```python
from build123d import *

# Parameters (mm, degrees)
BASE_DEPTH                = 5
ESQUISSE3_R               = 2
ESQUISSE3_W               = 65
ESQUISSE3_H               = 30
ENL_V_MAT_EXTRU_1_DEPTH   = 6
CONG_1_R                  = 3
PER_AGE_POUR_BILLES_REACH = 7
ESQUISSE6_R               = 2
ESQUISSE6_R_2             = 10.5
PER_AGE_POUR_PROFIL_REACH = 7
ESQUISSE8_R               = 3
ESQUISSE10_R              = 2
ENL_V_MAT_EXTRU_3_DEPTH   = 6


with BuildPart() as part:
    # Esquisse1 → Base (new body)
    with BuildSketch(Plane.XY):
        Polygon((0, 0), (-130, 0), (-154.748737342, 24.748737342), (-154.748737342, 244.748737342), (-130, 269.497474683), (0, 269.497474683), (24.748737342, 244.748737342), (24.748737342, 24.748737342), align=None)
    extrude(amount=BASE_DEPTH)

    # Esquisse3 → Enlèv. mat.-Extru.1 (cut, through all)
    with BuildSketch(Plane(origin=(0, 0, 0), x_dir=(-1, 0, 0), z_dir=(0, 0, -1))):
        with Locations((30, 45)):
            Circle(ESQUISSE3_R)
        with Locations((100, 45)):
            Circle(ESQUISSE3_R)
        with Locations((100, 224.497474683)):
            Circle(ESQUISSE3_R)
        with Locations((30, 224.497474683)):
            Circle(ESQUISSE3_R)
        Polygon((107, 0), (107, 20), (83, 20), (83, 45.5), (47, 45.5), (47, 20), (23, 20), (23, 0), align=None)
        Polygon((23, 269.497474683), (107, 269.497474683), (107, 249.497474683), (83, 249.497474683), (83, 223.997474683), (47, 223.997474683), (47, 249.497474683), (23, 249.497474683), align=None)
        with Locations((65, 199.497474683)):
            Rectangle(ESQUISSE3_W, ESQUISSE3_H)
        with Locations((65, 70)):
            Rectangle(ESQUISSE3_W, ESQUISSE3_H)
    extrude(amount=-ENL_V_MAT_EXTRU_1_DEPTH, mode=Mode.SUBTRACT)

    # Congé1
    cong_1_edges = [part.edges().sort_by_distance(p)[0] for p in [
        (0, 0, 2.5),
        (-130, 0, 2.5),
        (-154.748737342, 24.748737342, 2.5),
        (-154.748737342, 244.748737342, 2.5),
        (-130, 269.497474683, 2.5),
        (0, 269.497474683, 2.5),
        (24.748737342, 244.748737342, 2.5),
        (24.748737342, 24.748737342, 2.5),
        (-23, 249.497474683, 2.5),
        (-23, 269.497474683, 2.5),
        (-107, 269.497474683, 2.5),
        (-107, 249.497474683, 2.5),
        (-83, 249.497474683, 2.5),
        (-83, 223.997474683, 2.5),
        (-47, 223.997474683, 2.5),
        (-47, 249.497474683, 2.5),
        (-107, 0, 2.5),
        (-23, 0, 2.5),
        (-23, 20, 2.5),
        (-47, 20, 2.5),
        (-47, 45.5, 2.5),
        (-83, 45.5, 2.5),
        (-83, 20, 2.5),
        (-107, 20, 2.5),
    ]]
    fillet(cong_1_edges, radius=CONG_1_R)

    # Esquisse6 → Perçage pour billes (cut, up to next)
    with BuildSketch(Plane.XY.offset(5), mode=Mode.PRIVATE) as per_age_pour_billes_sk1:
        with Locations((-142, 55)):
            Circle(ESQUISSE6_R)
    per_age_pour_billes_tool1 = extrude(per_age_pour_billes_sk1.sketch, amount=-PER_AGE_POUR_BILLES_REACH, mode=Mode.PRIVATE) & part.part
    add(per_age_pour_billes_tool1.solids().sort_by_distance((-142, 55, 5))[0], mode=Mode.SUBTRACT)
    # Esquisse6 → Perçage pour billes (cut, up to next)
    with BuildSketch(Plane.XY.offset(5), mode=Mode.PRIVATE) as per_age_pour_billes_sk2:
        with Locations((-142, 85)):
            Circle(ESQUISSE6_R)
    per_age_pour_billes_tool2 = extrude(per_age_pour_billes_sk2.sketch, amount=-PER_AGE_POUR_BILLES_REACH, mode=Mode.PRIVATE) & part.part
    add(per_age_pour_billes_tool2.solids().sort_by_distance((-142, 85, 5))[0], mode=Mode.SUBTRACT)
    # Esquisse6 → Perçage pour billes (cut, up to next)
    with BuildSketch(Plane.XY.offset(5), mode=Mode.PRIVATE) as per_age_pour_billes_sk3:
        with Locations((-142, 70)):
            Circle(ESQUISSE6_R_2)
    per_age_pour_billes_tool3 = extrude(per_age_pour_billes_sk3.sketch, amount=-PER_AGE_POUR_BILLES_REACH, mode=Mode.PRIVATE) & part.part
    add(per_age_pour_billes_tool3.solids().sort_by_distance((-142, 70, 5))[0], mode=Mode.SUBTRACT)
    # Esquisse6 → Perçage pour billes (cut, up to next)
    with BuildSketch(Plane.XY.offset(5), mode=Mode.PRIVATE) as per_age_pour_billes_sk4:
        with Locations((-142, 214.497474683)):
            Circle(ESQUISSE6_R)
    per_age_pour_billes_tool4 = extrude(per_age_pour_billes_sk4.sketch, amount=-PER_AGE_POUR_BILLES_REACH, mode=Mode.PRIVATE) & part.part
    add(per_age_pour_billes_tool4.solids().sort_by_distance((-142, 214.497475, 5))[0], mode=Mode.SUBTRACT)
    # Esquisse6 → Perçage pour billes (cut, up to next)
    with BuildSketch(Plane.XY.offset(5), mode=Mode.PRIVATE) as per_age_pour_billes_sk5:
        with Locations((-142, 184.497474683)):
            Circle(ESQUISSE6_R)
    per_age_pour_billes_tool5 = extrude(per_age_pour_billes_sk5.sketch, amount=-PER_AGE_POUR_BILLES_REACH, mode=Mode.PRIVATE) & part.part
    add(per_age_pour_billes_tool5.solids().sort_by_distance((-142, 184.497475, 5))[0], mode=Mode.SUBTRACT)
    # Esquisse6 → Perçage pour billes (cut, up to next)
    with BuildSketch(Plane.XY.offset(5), mode=Mode.PRIVATE) as per_age_pour_billes_sk6:
        with Locations((-142, 199.497474683)):
            Circle(ESQUISSE6_R_2)
    per_age_pour_billes_tool6 = extrude(per_age_pour_billes_sk6.sketch, amount=-PER_AGE_POUR_BILLES_REACH, mode=Mode.PRIVATE) & part.part
    add(per_age_pour_billes_tool6.solids().sort_by_distance((-142, 199.497475, 5))[0], mode=Mode.SUBTRACT)
    # Esquisse6 → Perçage pour billes (cut, up to next)
    with BuildSketch(Plane.XY.offset(5), mode=Mode.PRIVATE) as per_age_pour_billes_sk7:
        with Locations((12, 55)):
            Circle(ESQUISSE6_R)
    per_age_pour_billes_tool7 = extrude(per_age_pour_billes_sk7.sketch, amount=-PER_AGE_POUR_BILLES_REACH, mode=Mode.PRIVATE) & part.part
    add(per_age_pour_billes_tool7.solids().sort_by_distance((12, 55, 5))[0], mode=Mode.SUBTRACT)
    # Esquisse6 → Perçage pour billes (cut, up to next)
    with BuildSketch(Plane.XY.offset(5), mode=Mode.PRIVATE) as per_age_pour_billes_sk8:
        with Locations((12, 184.497474683)):
            Circle(ESQUISSE6_R)
    per_age_pour_billes_tool8 = extrude(per_age_pour_billes_sk8.sketch, amount=-PER_AGE_POUR_BILLES_REACH, mode=Mode.PRIVATE) & part.part
    add(per_age_pour_billes_tool8.solids().sort_by_distance((12, 184.497475, 5))[0], mode=Mode.SUBTRACT)
    # Esquisse6 → Perçage pour billes (cut, up to next)
    with BuildSketch(Plane.XY.offset(5), mode=Mode.PRIVATE) as per_age_pour_billes_sk9:
        with Locations((12, 214.497474683)):
            Circle(ESQUISSE6_R)
    per_age_pour_billes_tool9 = extrude(per_age_pour_billes_sk9.sketch, amount=-PER_AGE_POUR_BILLES_REACH, mode=Mode.PRIVATE) & part.part
    add(per_age_pour_billes_tool9.solids().sort_by_distance((12, 214.497475, 5))[0], mode=Mode.SUBTRACT)
    # Esquisse6 → Perçage pour billes (cut, up to next)
    with BuildSketch(Plane.XY.offset(5), mode=Mode.PRIVATE) as per_age_pour_billes_sk10:
        with Locations((12, 85)):
            Circle(ESQUISSE6_R)
    per_age_pour_billes_tool10 = extrude(per_age_pour_billes_sk10.sketch, amount=-PER_AGE_POUR_BILLES_REACH, mode=Mode.PRIVATE) & part.part
    add(per_age_pour_billes_tool10.solids().sort_by_distance((12, 85, 5))[0], mode=Mode.SUBTRACT)
    # Esquisse6 → Perçage pour billes (cut, up to next)
    with BuildSketch(Plane.XY.offset(5), mode=Mode.PRIVATE) as per_age_pour_billes_sk11:
        with Locations((12, 70)):
            Circle(ESQUISSE6_R_2)
    per_age_pour_billes_tool11 = extrude(per_age_pour_billes_sk11.sketch, amount=-PER_AGE_POUR_BILLES_REACH, mode=Mode.PRIVATE) & part.part
    add(per_age_pour_billes_tool11.solids().sort_by_distance((12, 70, 5))[0], mode=Mode.SUBTRACT)
    # Esquisse6 → Perçage pour billes (cut, up to next)
    with BuildSketch(Plane.XY.offset(5), mode=Mode.PRIVATE) as per_age_pour_billes_sk12:
        with Locations((12, 199.497474683)):
            Circle(ESQUISSE6_R_2)
    per_age_pour_billes_tool12 = extrude(per_age_pour_billes_sk12.sketch, amount=-PER_AGE_POUR_BILLES_REACH, mode=Mode.PRIVATE) & part.part
    add(per_age_pour_billes_tool12.solids().sort_by_distance((12, 199.497475, 5))[0], mode=Mode.SUBTRACT)

    # Esquisse8 → Perçage pour profilé (cut, up to next)
    with BuildSketch(Plane.XY.offset(5), mode=Mode.PRIVATE) as per_age_pour_profil_sk1:
        with Locations((-118, 11)):
            Circle(ESQUISSE8_R)
    per_age_pour_profil_tool1 = extrude(per_age_pour_profil_sk1.sketch, amount=-PER_AGE_POUR_PROFIL_REACH, mode=Mode.PRIVATE) & part.part
    add(per_age_pour_profil_tool1.solids().sort_by_distance((-118, 11, 5))[0], mode=Mode.SUBTRACT)
    # Esquisse8 → Perçage pour profilé (cut, up to next)
    with BuildSketch(Plane.XY.offset(5), mode=Mode.PRIVATE) as per_age_pour_profil_sk2:
        with Locations((-118, 258.497474683)):
            Circle(ESQUISSE8_R)
    per_age_pour_profil_tool2 = extrude(per_age_pour_profil_sk2.sketch, amount=-PER_AGE_POUR_PROFIL_REACH, mode=Mode.PRIVATE) & part.part
    add(per_age_pour_profil_tool2.solids().sort_by_distance((-118, 258.497475, 5))[0], mode=Mode.SUBTRACT)
    # Esquisse8 → Perçage pour profilé (cut, up to next)
    with BuildSketch(Plane.XY.offset(5), mode=Mode.PRIVATE) as per_age_pour_profil_sk3:
        with Locations((-12, 258.497474683)):
            Circle(ESQUISSE8_R)
    per_age_pour_profil_tool3 = extrude(per_age_pour_profil_sk3.sketch, amount=-PER_AGE_POUR_PROFIL_REACH, mode=Mode.PRIVATE) & part.part
    add(per_age_pour_profil_tool3.solids().sort_by_distance((-12, 258.497475, 5))[0], mode=Mode.SUBTRACT)
    # Esquisse8 → Perçage pour profilé (cut, up to next)
    with BuildSketch(Plane.XY.offset(5), mode=Mode.PRIVATE) as per_age_pour_profil_sk4:
        with Locations((-12, 11)):
            Circle(ESQUISSE8_R)
    per_age_pour_profil_tool4 = extrude(per_age_pour_profil_sk4.sketch, amount=-PER_AGE_POUR_PROFIL_REACH, mode=Mode.PRIVATE) & part.part
    add(per_age_pour_profil_tool4.solids().sort_by_distance((-12, 11, 5))[0], mode=Mode.SUBTRACT)

    # Esquisse10 → Enlèv. mat.-Extru.3 (cut, through all)
    with BuildSketch(Plane.XY.offset(5)):
        with Locations((-97, 174.497474683)):
            Circle(ESQUISSE10_R)
        with Locations((-97, 148.497474683)):
            Circle(ESQUISSE10_R)
        with Locations((-33, 148.497474683)):
            Circle(ESQUISSE10_R)
        with Locations((-33, 174.497474683)):
            Circle(ESQUISSE10_R)
        with Locations((-33, 121)):
            Circle(ESQUISSE10_R)
        with Locations((-33, 95)):
            Circle(ESQUISSE10_R)
        with Locations((-97, 121)):
            Circle(ESQUISSE10_R)
        with Locations((-97, 95)):
            Circle(ESQUISSE10_R)
    extrude(amount=-ENL_V_MAT_EXTRU_3_DEPTH, mode=Mode.SUBTRACT)


solid = part.part
```
Input: part model. Units: mm. Frame: model coordinates. A direction names the side the tool comes from. Give positions to 0.01 mm unless a question says otherwise; leave off trailing zeros. Order: outer loops, then holes, each group sorted by start corner. A loop starts at its lowest first (then second) coordinate and runs counter-clockwise, first axis right, second up. Notation, with made-up numbers: M 3,-27.5 L 50,-27.5 A6 ccw 50,-21.5 Z; hole C 43.5,63 d3. An arc over 180 degrees is marked long. Return JSON: item names as keys, results as strings.
1) Mould query, pull axis X, two halves, no side actions, for faces 1 (the face through (-10, 0, 2)), 2 (the face through (-14.4, 9.2, 2.5)), 3 (the face through (-142.5, 257, 2.5)). Classes: released by +X, released by -X, zero draft, split by the parting line, or undercut.
Taken from the geometry:
{"face 1": "zero draft", "face 2": "undercut", "face 3": "released by -X"}
2) Contact query for flat-ended pins moving along their axis: pin 1 (2.5 mm diameter, centred on x = -76.5, z = 1.5, fed in from -Y); pin 2 (8 mm diameter, centred on x = -12, y = 11, fed in from -Z); pin 3 (3 mm diameter, centred on x = 6.5, z = 3.5, fed in from +Y); pin 4 (1.5 mm diameter, centred on x = -53, z = 2.5, fed in from +Y). Output: stop coordinate, or through.
Taken from the geometry:
{"pin 1": "stops at y = 45.5", "pin 2": "stops at z = 0", "pin 3": "stops at y = 264.5", "pin 4": "stops at y = 224"}
3) Section query A-A on y = 11. Output: boundary loops of the cut face in (x, z), and give its area (3 significant figures).
Taken from the geometry:
{"outline": "M -141,0 L -121,0 L -121,5 L -141,5 Z; M -115,0 L -107,0 L -107,5 L -115,5 Z; M -23,0 L -15,0 L -15,5 L -23,5 Z; M -9,0 L 11,0 L 11,5 L -9,5 Z", "area": "280 mm2"}
4) Access query for faces 4 (the face through (-47, 33, 2)), 5 (the face through (-32.5, 199, 2)), 6 (the face through (-64, 137, 5)), 7 (the face through (-95, 249.497, 2)). Directions: +Z, -Z, +X, -X, +Y, -Y. A direction counts if a zero-diameter tool reaches every point of the face in a straight line with its end or side. Return the directions, or none.
Taken from the geometry:
{"face 4": "+Z, -Z, -Y", "face 5": "+Z, -Z", "face 6": "+Z, +X, -X, +Y, -Y", "face 7": "+Z, -Z, +Y"}
5) Section query C-C on z = 2. Count the separate pieces of the cut face and the enclosed holes in it, and give its area (3 significant figures).
Taken from the geometry:
{"separate pieces": "1", "enclosed holes": "30", "area": "36,300 mm2"}
6) Section query B-B on y = 196. Output: boundary loops of the cut face in (x, z).
Taken from the geometry:
{"outline": "M -154.75,0 L -151.9,0 L -151.9,5 L -154.75,5 Z; M -132.1,0 L -97.5,0 L -97.5,5 L -132.1,5 Z; M -32.5,0 L 2.1,0 L 2.1,5 L -32.5,5 Z; M 21.9,0 L 24.75,0 L 24.75,5 L 21.9,5 Z"}
7) Line query: L1, parallel to Y at x = -89.5, z = 3; L2, parallel to X at y = 247, z = 3.2; L3, parallel to Y at x = -52, z = 3.05. Output: solid intervals per line, ascending. Write a range as [from, to].
Taken from the geometry:
{"L1": "y = [20, 55], [85, 184.5], [214.5, 249.5]", "L2": "x = [-152.5, -83.04], [-46.96, 22.5]", "L3": "y = [45.5, 55], [85, 184.5], [214.5, 224]"}
